Verification items for the finished model (mm, model axes). Face numbers are marked on the shaded views. A direction names the side the tool comes from. Round coordinates to 2 decimals unless told otherwise and drop trailing zeros. Loops run counter-clockwise (first coordinate to the right, second up) from the corner with the lowest first, then second, coordinate; pieces in that order, holes last. Notation, with made-up numbers: (-10, -26) - (1, -26) arc R20 ccw to (1, 10) - close; hole circle Ø6 at (58, 43). An arc over 180 degrees is marked (long way). Use CSV: the item, a comma, the result in double quotes.
```python
from build123d import *

# Parameters (mm, degrees)
EXTRUDE3_DEPTH = 15.24
EXTRUDE4_DEPTH = 6.477
SKETCH7_R      = 7.8994
EXTRUDE5_DEPTH = 4.0132
SKETCH8_R      = 2.2987
EXTRUDE6_DEPTH = 4.2926
SKETCH9_R      = 4.4196
EXTRUDE7_DEPTH = 4.4196
SKETCH10_R     = 4.7244
SKETCH10_R_2   = 1.905
SKETCH10_R_3   = 1.179287719
SKETCH10_R_4   = 2.031992692
EXTRUDE8_DEPTH = 17.5768


with BuildPart() as part:
    # Sketch4 → Extrude3 (new body)
    with BuildSketch(Plane.XY):
        with BuildLine():
            Line((-42.343481517, -2.990600597), (-42.343481517, 17.964399403))
            ThreePointArc((-42.343481517, 17.964399403), (-41.413545547, 20.209463433), (-39.168481517, 21.139399403))
            Line((-39.168481517, 21.139399403), (-15.038481517, 21.139399403))
            Line((-15.038481517, 21.139399403), (-15.038481517, 18.236569756))
            ThreePointArc((-15.038481517, 18.236569756), (-14.108545547, 15.991505726), (-11.863481517, 15.061569756))
            Line((-11.863481517, 15.061569756), (9.257081626, 15.061569756))
            ThreePointArc((9.257081626, 15.061569756), (11.502145656, 15.991505726), (12.432081626, 18.236569756))
            Line((12.432081626, 18.236569756), (12.432081626, 22.681569756))
            Line((12.432081626, 22.681569756), (52.437081626, 22.681569756))
            ThreePointArc((52.437081626, 22.681569756), (54.682145656, 21.751633786), (55.612081626, 19.506569756))
            Line((55.612081626, 19.506569756), (55.612081626, -9.945714332))
            ThreePointArc((55.612081626, -9.945714332), (56.542017596, -12.190778362), (58.787081626, -13.120714332))
            Line((58.787081626, -13.120714332), (61.618454053, -13.120714332))
            Line((61.618454053, -13.120714332), (61.618454053, -19.76149571))
            Line((61.618454053, -19.76149571), (12.432081626, -19.76149571))
            Line((12.432081626, -19.76149571), (12.432081626, -17.323430244))
            ThreePointArc((12.432081626, -17.323430244), (11.502145656, -15.078366214), (9.257081626, -14.148430244))
            Line((9.257081626, -14.148430244), (-18.530518374, -14.148430244))
            ThreePointArc((-18.530518374, -14.148430244), (-20.775582404, -15.078366214), (-21.705518374, -17.323430244))
            Line((-21.705518374, -17.323430244), (-21.705518374, -19.76149571))
            Line((-21.705518374, -19.76149571), (-40.618560355, -19.76149571))
            Line((-40.618560355, -19.76149571), (-40.618560355, -13.120714332))
            Line((-40.618560355, -13.120714332), (-35.040518374, -13.120714332))
            ThreePointArc((-35.040518374, -13.120714332), (-32.795454344, -12.190778362), (-31.865518374, -9.945714332))
            Line((-31.865518374, -9.945714332), (-31.865518374, -9.340600597))
            ThreePointArc((-31.865518374, -9.340600597), (-32.795454344, -7.095536567), (-35.040518374, -6.165600597))
            Line((-35.040518374, -6.165600597), (-39.168481517, -6.165600597))
            ThreePointArc((-39.168481517, -6.165600597), (-41.413545547, -5.235664628), (-42.343481517, -2.990600597))
        make_face()
    extrude(amount=EXTRUDE3_DEPTH)

    # Sketch1 → Extrude4 (cut)
    with BuildSketch(Plane.XY):
        with BuildLine():
            Line((-35.993481517, 11.614399403), (-35.993481517, 2.089399403))
            ThreePointArc((-35.993481517, 2.089399403), (-35.063545547, -0.155664628), (-32.818481517, -1.085600597))
            Line((-32.818481517, -1.085600597), (-26.785518374, -1.085600597))
            Line((-26.785518374, -1.085600597), (-26.785518374, -5.893430244))
            ThreePointArc((-26.785518374, -5.893430244), (-25.855582404, -8.138494274), (-23.610518374, -9.068430244))
            Line((-23.610518374, -9.068430244), (17.512081626, -9.068430244))
            Line((17.512081626, -9.068430244), (17.512081626, -12.243430244))
            ThreePointArc((17.512081626, -12.243430244), (18.442017596, -14.488494274), (20.687081626, -15.418430244))
            Line((20.687081626, -15.418430244), (46.087081626, -15.418430244))
            ThreePointArc((46.087081626, -15.418430244), (48.332145656, -14.488494274), (49.262081626, -12.243430244))
            Line((49.262081626, -12.243430244), (49.262081626, 13.156569756))
            ThreePointArc((49.262081626, 13.156569756), (48.332145656, 15.401633786), (46.087081626, 16.331569756))
            Line((46.087081626, 16.331569756), (20.687081626, 16.331569756))
            ThreePointArc((20.687081626, 16.331569756), (18.442017596, 15.401633786), (17.512081626, 13.156569756))
            Line((17.512081626, 13.156569756), (17.512081626, 9.981569756))
            Line((17.512081626, 9.981569756), (-20.118481517, 9.981569756))
            Line((-20.118481517, 9.981569756), (-20.118481517, 11.614399403))
            ThreePointArc((-20.118481517, 11.614399403), (-21.048417487, 13.859463433), (-23.293481517, 14.789399403))
            Line((-23.293481517, 14.789399403), (-32.818481517, 14.789399403))
            ThreePointArc((-32.818481517, 14.789399403), (-35.063545547, 13.859463433), (-35.993481517, 11.614399403))
        make_face()
    extrude(amount=EXTRUDE4_DEPTH, mode=Mode.SUBTRACT)

    # Sketch7 → Extrude5 (cut)
    with BuildSketch(Plane(origin=(0, 0, 6.477), x_dir=(-1, 0, 0), z_dir=(0, 0, -1))):
        with Locations((-33.387081626, 0.456569756)):
            Circle(SKETCH7_R)
    extrude(amount=-EXTRUDE5_DEPTH, mode=Mode.SUBTRACT)

    # Sketch8 → Extrude6 (cut)
    with BuildSketch(Plane(origin=(0, 0, 6.477), x_dir=(-1, 0, 0), z_dir=(0, 0, -1))):
        with Locations((-12.305081626, 0.456569756)):
            Circle(SKETCH8_R)
        with Locations((2.477718374, 0.456569756)):
            Circle(SKETCH8_R)
        with Locations((17.260518374, 0.456569756)):
            Circle(SKETCH8_R)
    extrude(amount=-EXTRUDE6_DEPTH, mode=Mode.SUBTRACT)

    # Sketch9 → Extrude7 (cut)
    with BuildSketch(Plane(origin=(0, 0, 6.477), x_dir=(-1, 0, 0), z_dir=(0, 0, -1))):
        with Locations((28.055981517, 6.851899403)):
            Circle(SKETCH9_R)
    extrude(amount=-EXTRUDE7_DEPTH, mode=Mode.SUBTRACT)

    # Sketch10 → Extrude8 (cut, symmetric)
    with BuildSketch(Plane(origin=(0, 0, 10.4902), x_dir=(-1, 0, 0), z_dir=(0, 0, -1))):
        with Locations((-33.387081626, 0.456569756)):
            Circle(SKETCH10_R)
        with Locations((-52.287415303, -15.678066597)):
            Circle(SKETCH10_R_2)
        with Locations((28.055981517, 6.851899403)):
            Circle(SKETCH10_R_3)
        with Locations((37.474326825, 16.270244711)):
            Circle(SKETCH10_R_2)
        with Locations((-13.846294556, 13.596903192)):
            Circle(SKETCH10_R_2)
        with Locations((-13.846294556, -12.683763681)):
            Circle(SKETCH10_R_2)
        with Locations((27.221195322, -14.622613425)):
            Circle(SKETCH10_R_4)
        with Locations((-50.814973838, 17.884461968)):
            Circle(SKETCH10_R_2)
        with Locations((16.452694446, 13.596903192)):
            Circle(SKETCH10_R_2)
    extrude(amount=EXTRUDE8_DEPTH, both=True, mode=Mode.SUBTRACT)


solid = part.part
```
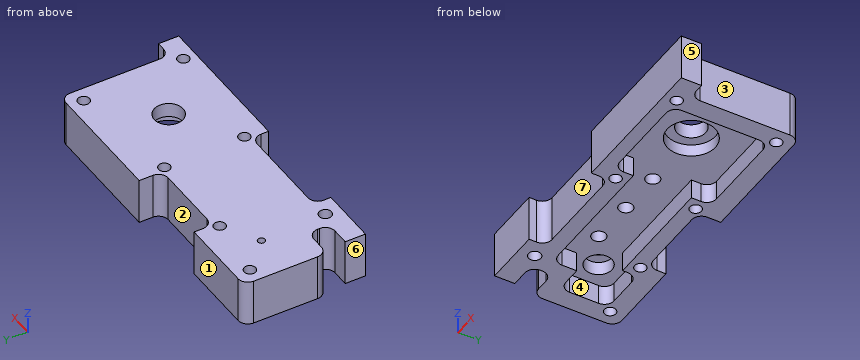
1) Mould release check, pull along X, two halves, no side actions. Record for the marked faces 5, 6 and 7: +X half, -X half, draft (parallel to the pull), parting line (faces both ways), or undercut.
Returned:
face 5,"+X half"
face 6,"-X half"
face 7,"undercut"
2) Gauge pin test, flat ends, axial feed: pin 1 Ø8 at (x, y) = (31, 2) entering from -Z; pin 2 Ø1.4 at (x, y) = (-18, 1.5) entering from -Z; pin 3 Ø1.5 at (x, z) = (5, 9) entering from -Y; pin 4 Ø3 at (x, y) = (13.85, -12.68) entering from -Z. Record the tip position at first contact, or that the pin passes through.
Returned:
pin 1,"stops at z = 10.49"
pin 2,"stops at z = 10.77"
pin 3,"stops at y = -14.15"
pin 4,"passes through"
3) Cross-section at B-B, the plane x = 3.5. Record the cut outline in (y, z), then the cut area to 3 significant figures.
Returned:
outline,"(-14.15, 0) - (-9.07, 0) - (-9.07, 6.48) - (9.98, 6.48) - (9.98, 0) - (15.06, 0) - (15.06, 15.24) - (-14.15, 15.24) - close"
area,"322 mm²"
4) Access from +Z, -Z, +X, -X, +Y, -Y to the whole of each face (thin tool, end or side, straight path). Record for the marked faces 1, 2, 3 and 4.
Returned:
face 1,"+Z, -Z, -X, +Y"
face 2,"+Z, -Z, +Y"
face 3,"+Z, -Z, +X, +Y"
face 4,"-Z"
5) Cross-section at A-A, the plane x = 31. Record the cut outline in (y, z).
Returned:
outline,"(-19.76, 0) - (-15.42, 0) - (-15.42, 6.48) - (-7.07, 6.48) - (-7.07, 10.49) - (-3.62, 10.49) - (-3.62, 15.24) - (-19.76, 15.24) - close; (4.53, 10.49) - (7.99, 10.49) - (7.99, 6.48) - (16.33, 6.48) - (16.33, 0) - (22.68, 0) - (22.68, 15.24) - (4.53, 15.24) - close"
6) Cross-section at C-C, the plane z = 9. Count the separate pieces of the cut face and the enclosed holes in it, then the cut area to 3 significant figures.
Returned:
separate pieces,"1"
enclosed holes,"12"
area,"3,290 mm²"
7) Thickness scan on probe 1 along Y at (x, z) = (44, 4.75); probe 2 along X at (y, z) = (9.5, 3.5); probe 3 along X at (y, z) = (-18, 8.75). Record the ranges inside material, lowest first. Write a range as [from, to].
Returned:
probe 1,"y = [-19.76, -15.42], [16.33, 22.68]"
probe 2,"x = [-42.34, -35.99], [49.26, 55.61]"
probe 3,"x = [-40.62, -21.71], [12.43, 61.62]"
